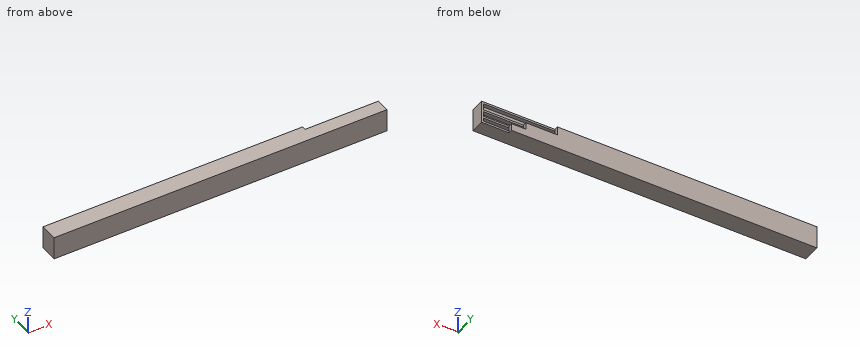
```python
from build123d import *

# Parameters (mm, degrees)
SKETCH1_W           = 506
SKETCH1_H           = 34.5
BOSS_EXTRUDE1_DEPTH = 15
SKETCH3_W           = 506
SKETCH3_H           = 34.5
SKETCH3_W_2         = 500
SKETCH3_H_2         = 10
SKETCH3_H_3         = 5
SKETCH3_H_4         = 7.5
BOSS_EXTRUDE2_DEPTH = 6
BOSS_EXTRUDE3_DEPTH = 6


with BuildPart() as part:
    # Sketch1 → Boss-Extrude1 (new body)
    with BuildSketch(Plane(origin=(0, 0, 0), x_dir=(1, 0, 0), z_dir=(0, 1, 0))):
        with Locations((250, -9.25)):
            Rectangle(SKETCH1_W, SKETCH1_H)
    extrude(amount=-BOSS_EXTRUDE1_DEPTH)

    # Sketch3 → Boss-Extrude2 (add)
    with BuildSketch(Plane(origin=(0, 0, 0), x_dir=(1, 0, 0), z_dir=(0, 1, 0))):
        with Locations((250, -9.25)):
            Rectangle(SKETCH3_W, SKETCH3_H)
        with Locations((250, -18.5)):
            Rectangle(SKETCH3_W_2, SKETCH3_H_2, mode=Mode.SUBTRACT)
        with Locations((250, 2.5)):
            Rectangle(SKETCH3_W_2, SKETCH3_H_3, mode=Mode.SUBTRACT)
        with Locations((250, -6.75)):
            Rectangle(SKETCH3_W_2, SKETCH3_H_4, mode=Mode.SUBTRACT)
    extrude(amount=BOSS_EXTRUDE2_DEPTH)

    # Sketch4 → Boss-Extrude3 (add)
    with BuildSketch(Plane(origin=(0, 6, 0), x_dir=(1, 0, 0), z_dir=(0, 1, 0))):
        Polygon((461.264937975, 8), (461.264937975, -3), (439.515598099, -3), (439.515598099, -13.5), (391.45657289, -13.5), (391.45657289, -26.5), (-3, -26.5), (-3, 8), align=None)
    extrude(amount=BOSS_EXTRUDE3_DEPTH)


solid = part.part
```
Here's how the part is built. I have some questions about the finished solid (model axes, mm). Round coordinates to 2 decimals unless told otherwise and drop trailing zeros. Write each loop counter-clockwise with the first axis right and the second up, starting at its lowest first coordinate (ties: lowest second). Pieces come first, ordered by that corner, then holes.
Q1. If we section it at A-A on x = 454: Write out the boundary of the cut face in (y, z).
Q2. Please list where these lines run through material, in increasing order: probe 1 along Z at (x, y) = (248.5, 2); probe 2 along Y at (x, z) = (362, 5); probe 3 along X at (y, z) = (0.5, -4.5).
Q3. Will this pin go through, and if not, where does the flat tip stop? P1, Ø10.5, axis at x = 447.5, z = 13, coming from the +Y side.
Q4. If we section it at B-B on x = 159.5: Write out the boundary of the cut face in (y, z), plus the area to 4 significant figures.
Answer below:
1. outline: (-15, -8) - (12, -8) - (12, 3) - (0, 3) - (0, 10.5) - (6, 10.5) - (6, 13.5) - (0, 13.5) - (0, 23.5) - (6, 23.5) - (6, 26.5) - (-15, 26.5) - close; hole (0, -5) - (6, -5) - (6, 0) - (0, 0) - close
2. probe 1: z = -8 to -5, 0 to 3, 10.5 to 13.5, 23.5 to 26.5
2. probe 2: y = -15 to 0, 6 to 12
2. probe 3: x = -3 to 0, 500 to 503
3. P1: stops at y = 6
4. outline: (-15, -8) - (12, -8) - (12, 26.5) - (-15, 26.5) - close; hole (0, -5) - (6, -5) - (6, 0) - (0, 0) - close; hole (0, 3) - (6, 3) - (6, 10.5) - (0, 10.5) - close; hole (0, 13.5) - (6, 13.5) - (6, 23.5) - (0, 23.5) - close
4. area: 796.5 mm2
